```python
from build123d import *

# Parameters (mm, degrees)
SKETCH1_R                 = 14
BOSS_EXTRUDE1_DEPTH       = 100
SKETCH2_R                 = 11
SKETCH2_R_2               = 3
BOSS_EXTRUDE2_DEPTH       = 7
SKETCH2_3_R               = 3
BOSS_EXTRUDE3_DEPTH       = 23
BOSS_EXTRUDE4_START       = 5
SKETCH2_4_R               = 18
SKETCH2_4_R_2             = 14
SKETCH2_4_R_3             = 11
BOSS_EXTRUDE4_DEPTH       = 5
M3X0_5_TAPPED_HOLE1_D     = 2.5
M3X0_5_TAPPED_HOLE1_DEPTH = 5


with BuildPart() as part:
    # Sketch1 → Boss-Extrude1 (new body)
    with BuildSketch(Plane.XY):
        Circle(SKETCH1_R)
    extrude(amount=BOSS_EXTRUDE1_DEPTH)

    # Sketch2 → Boss-Extrude2 (add)
    # profile 1 of 2: a face of its own
    with BuildSketch(Plane(origin=(0, 0, 0), x_dir=(-1, 0, 0), z_dir=(0, 0, -1))):
        Circle(SKETCH2_R)
        Circle(SKETCH2_R_2, mode=Mode.SUBTRACT)
    # profile 2 of 2: a face of its own
    with BuildSketch(Plane(origin=(0, 0, 0), x_dir=(-1, 0, 0), z_dir=(0, 0, -1))):
        Circle(SKETCH2_R_2)
    extrude(amount=BOSS_EXTRUDE2_DEPTH)

    # Sketch2<3> → Boss-Extrude3 (add)
    with BuildSketch(Plane(origin=(0, 0, 0), x_dir=(-1, 0, 0), z_dir=(0, 0, -1))):
        Circle(SKETCH2_3_R)
    extrude(amount=BOSS_EXTRUDE3_DEPTH)

    # Sketch2<4> → Boss-Extrude4 (add)
    # profile 1 of 2: a face of its own
    with BuildSketch(Plane(origin=(0, 0, 0), x_dir=(-1, 0, 0), z_dir=(0, 0, -1)).offset(BOSS_EXTRUDE4_START)):
        Circle(SKETCH2_4_R)
        Circle(SKETCH2_4_R_2, mode=Mode.SUBTRACT)
    # profile 2 of 2: a face of its own
    with BuildSketch(Plane(origin=(0, 0, 0), x_dir=(-1, 0, 0), z_dir=(0, 0, -1)).offset(BOSS_EXTRUDE4_START)):
        Circle(SKETCH2_4_R_2)
        Circle(SKETCH2_4_R_3, mode=Mode.SUBTRACT)
    extrude(amount=-BOSS_EXTRUDE4_DEPTH)

    # M3x0.5 Tapped Hole1
    with Locations(Plane(origin=(0, 0, -5), x_dir=(-1, 0, 0), z_dir=(0, 0, -1))):
        with Locations((0, 14), (14, 0), (0, -14), (-14, 0)):
            Hole(M3X0_5_TAPPED_HOLE1_D / 2, depth=M3X0_5_TAPPED_HOLE1_DEPTH)


solid = part.part
```
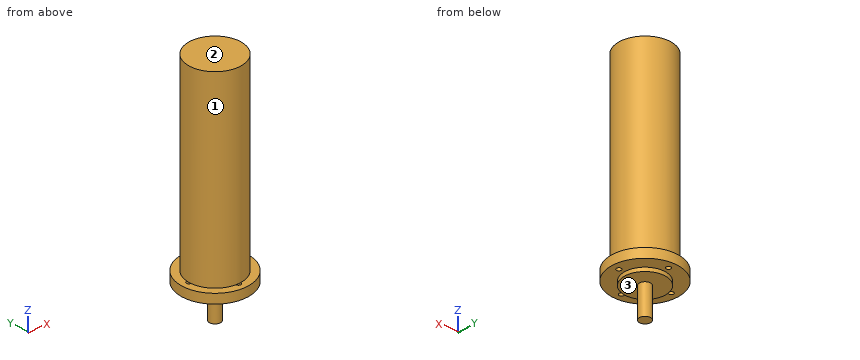
Model file for the job. Use its own axes, mm. Face numbers are marked on the shaded views. A direction names the side the tool comes from. Give positions to 0.01 mm unless a question says otherwise; leave off trailing zeros. Loops run counter-clockwise (first coordinate to the right, second up) from the corner with the lowest first, then second, coordinate; pieces in that order, holes last. Notation, with made-up numbers: (-29.75, 9.25) - (24.25, 9.25) arc R19 cw to (24.25, 25.25) - close; hole circle Ø10 at (2.5, 0). An arc over 180 degrees is marked (long way). One line per item, written item: value. Start each with the question number.
1. Slice it at B-B (z = -12). List the corners of the cut face in (x, y).
2. Slice it at A-A (x = 0). List the corners of the cut face in (y, z), plus the area to 4 significant figures.
3. Which spindle directions (+Z, -Z, +X, -X, +Y, -Y) get a long thin tool onto all of the face, cutting with end or side? Do the marked faces 1, 2 and 3. Say none if no direction does.
4. Pin check, flat tips, straight feed: pin 1 (4 mm diameter, centred on x = 0, y = 14, fed in from -Z); pin 2 (4 mm diameter, centred on y = -11, z = 71, fed in from +X); pin 3 (5 mm diameter, centred on y = 2, z = 17.5, fed in from -X). Stop position of each tip, or through.
5. Slice it at C-C (x = 5). List the corners of the cut face in (y, z), plus the area to 3 significant figures.
6. Slice it at D-D (z = 59). List the corners of the cut face in (x, y).
7. Probe L1, parallel to Y at x = 0, z = -1; L2, parallel to Z at x = 8, y = -10.5; L3, parallel to Z at x = 12, y = 12. List the from-to ranges inside material, lowest first. Write a range as from..to.
Solution:
1. outline: circle Ø6 at (0, 0)
2. outline: (-18, -5) - (-15.25, -5) - (-15.25, 0) - (-18, 0) - close; (-14, 0) - (-12.75, 0) - (-12.75, -5) - (-11, -5) - (-11, -7) - (-3, -7) - (-3, -23) - (3, -23) - (3, -7) - (11, -7) - (11, -5) - (12.75, -5) - (12.75, 0) - (14, 0) - (14, 100) - (-14, 100) - close; (15.25, -5) - (18, -5) - (18, 0) - (15.25, 0) - close
2. area: 3,095 mm^2
3. face 1: +Z
3. face 2: +Z, +X, -X, +Y, -Y
3. face 3: -Z
4. pin 1: stops at z = -5
4. pin 2: stops at x = 10.72
4. pin 3: stops at x = -14
5. outline: (-17.29, -5) - (-9.8, -5) - (-9.8, -7) - (9.8, -7) - (9.8, -5) - (17.29, -5) - (17.29, 0) - (13.08, 0) - (13.08, 100) - (-13.08, 100) - (-13.08, 0) - (-17.29, 0) - close
5. area: 2,830 mm^2
6. outline: circle Ø28 at (0, 0)
7. L1: y = -18..-15.25, -12.75..12.75, 15.25..18
7. L2: z = -5..100
7. L3: z = -5..0
